Read the model definition and answer for the solid it produces. Units are mm, in the model's axes. A direction names the side the tool comes from. Coordinates: 2 decimals unless noted, no trailing zeros. Loops run counter-clockwise (first coordinate to the right, second up) from the corner with the lowest first, then second, coordinate; pieces in that order, holes last. Notation, with made-up numbers: M -33.5,-26 L 2.5,-26 A27 cw 2.5,4 Z; hole C 8.25,46.5 d10. An arc over 180 degrees is marked long. Use one line per item in the form item = value. Start each with the question number.
1. The part is cut by section A-A (x = 0). Give the vertices of the cut face in (y, z).
2. The part is cut by section C-C (z = -3.25). Give the vertices of the cut face in (x, y), plus the area to 3 significant figures.
3. A tool of negligible diameter and unlimited length cuts with its end or side. For faces 1 (the flat face through (0, 0, -11.43)), 2 (the cylindrical face through (-1.89, -1.45, -5.63)), from which of +Z, -Z, +X, -X, +Y, -Y can it reach the whole face along a straight path? Write none if from no direction.
4. Flat-ended cylindrical pins translate along their axes: pin 1 (1.5 mm diameter, centred on x = -1.5, z = -5.5, fed in from -Y); pin 2 (5 mm diameter, centred on x = 0, z = -6, fed in from -Y). Find the tip coordinate at first contact, or state that the pin passes through.
5. Find the intervals of material crossed by probe 1 along Y at (x, z) = (-2.5, 0.5); probe 2 along Y at (x, z) = (-2, -5.5); probe 3 along Z at (x, y) = (3, 0.25), in increasing order. Write a range as [from, to].
from build123d import *

# Parameters (mm, degrees)
SKETCH1_R           = 5.0038
BOSS_EXTRUDE1_DEPTH = 1.6002
SKETCH2_R           = 2.38125
BOSS_EXTRUDE2_DEPTH = 11.43
FILLET1_R           = 2.54


with BuildPart() as part:
    # Sketch1 → Boss-Extrude1 (new body)
    with BuildSketch(Plane.XY):
        Circle(SKETCH1_R)
    extrude(amount=BOSS_EXTRUDE1_DEPTH)

    # Sketch2 → Boss-Extrude2 (add)
    with BuildSketch(Plane.XY):
        Circle(SKETCH2_R)
    extrude(amount=-BOSS_EXTRUDE2_DEPTH)

    # Fillet1
    # the kernel refuses this fillet: 2.54 mm, written as the material it takes off along each edge
    with BuildSketch(Plane(origin=(0, 0, 1.6002), x_dir=(1, 0, 0), z_dir=(0, -1, 0))) as fillet1_piece_1:
        with BuildLine():
            CenterArc((2.644059345, -2.54), FILLET1_R, 21.715617283, 68.284382717)
            Line((2.644059345, 0), (2.644059345, 0.0508))
            Line((2.644059345, 0.0508), (5.0038, 0.0508))
            Line((5.0038, 0.0508), (5.0546, 0))
            ThreePointArc((5.0546, 0), (5.0546, -0.8001), (5.050994813, -1.581404))
            Line((5.050994813, -1.581404), (5.0038, -1.6002))
        make_face()
    revolve(axis=Axis((0, 0, 1.6002), (0, 0, 1)), mode=Mode.SUBTRACT)


solid = part.part
Computed values:
q1.outline = M -5,0 L -2.38,0 L -2.38,-11.43 L 2.38,-11.43 L 2.38,0 L 5,0 A2.54 ccw 2.64,1.6 L -2.64,1.6 A2.54 ccw Z
q2.outline = C 0,0 d4.76
q2.area = 17.8 mm²
q3.face_1 = -Z, +X, -X, +Y, -Y
q3.face_2 = -Z
q4.pin_1 = -2.26
q4.pin_2 = -2.38
q5.probe_1 = [-4.02, 4.02]
q5.probe_2 = [-1.29, 1.29]
q5.probe_3 = [0, 1.57]
